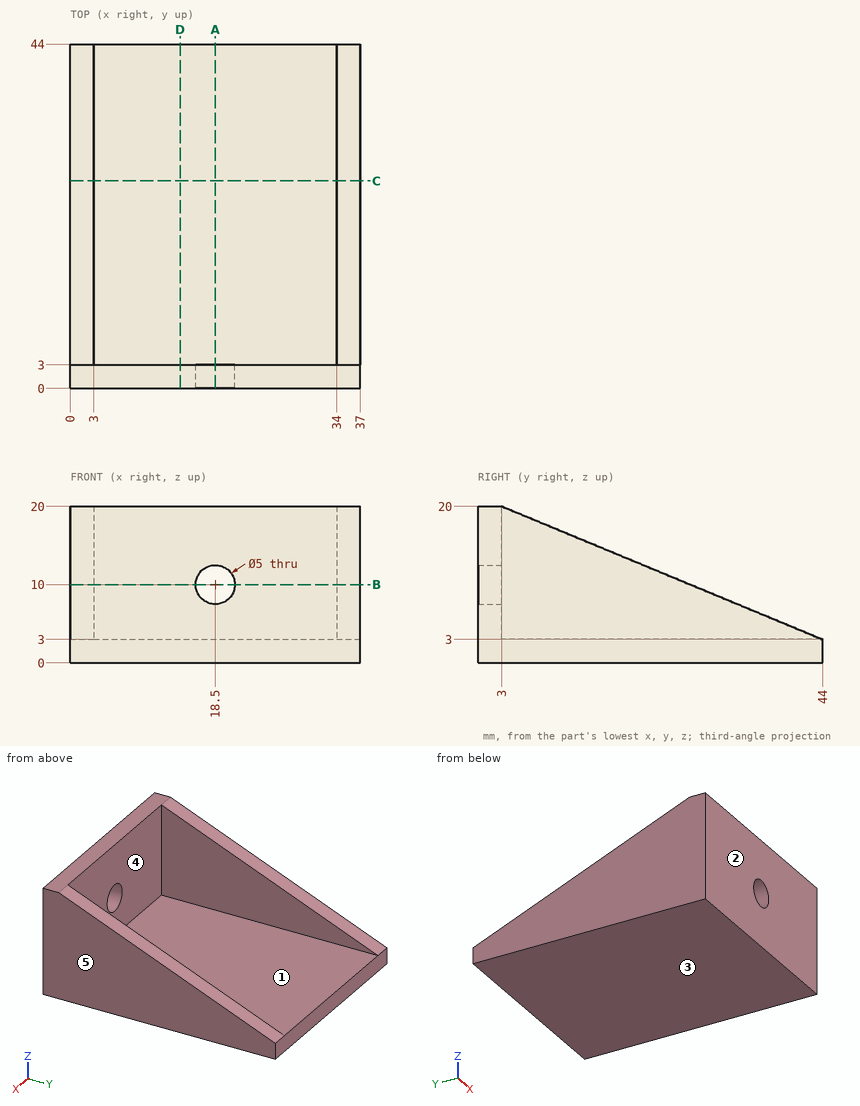
Source: three-view drawing plus pictorial views. Frame: mm from the lowest corner of the part. A direction names the side the tool comes from. Round coordinates to 2 decimals unless told otherwise and drop trailing zeros. Loops run counter-clockwise (first coordinate to the right, second up) from the corner with the lowest first, then second, coordinate; pieces in that order, holes last.
Q1. Section D-D on x = 14. Return loops of the section in (y, z), plus the area to 3 significant figures.
Q2. Section C-C on y = 26.5. Return loops of the section in (x, z), plus the area to 3 significant figures.
Q3. Section A-A on x = 18.5. Return loops of the section in (y, z), plus the area to 3 significant figures.
Q4. Section B-B on z = 10. Return loops of the section in (x, y), plus the area to 3 significant figures.
Q5. Access query for the marked faces 1 and 2. Directions: +Z, -Z, +X, -X, +Y, -Y. A direction counts if a zero-diameter tool reaches every point of the face in a straight line with its end or side. Return the directions, or none.
Q6. Pin query (flat end, axial travel): P1, Ø1.5, axis at x = 7, y = 39, coming from the +Z side; P2, Ø5, axis at x = 16, z = 15, coming from the +Y side. Return the tip coordinate at first contact, or that it passes through.
Q7. Pull-direction query (X, two-part tool) for the marked faces 3, 4 and 5; classes: released by +X, released by -X, zero draft, split by the parting line, or undercut.
Q8. Material intervals for L1, parallel to X at y = 39.5, z = 3.25; L2, parallel to Z at x = 18.5, y = 0.75; L3, parallel to Y at x = 20.5, z = 12.25, sorted ascending.
Evaluation:
1. outline: (0, 0) - (44, 0) - (44, 3) - (3, 3) - (3, 20) - (0, 20) - close
1. area: 183 mm2
2. outline: (0, 0) - (37, 0) - (37, 10.26) - (34, 10.26) - (34, 3) - (3, 3) - (3, 10.26) - (0, 10.26) - close
2. area: 155 mm2
3. outline: (0, 0) - (44, 0) - (44, 3) - (3, 3) - (3, 7.5) - (0, 7.5) - close; (0, 12.5) - (3, 12.5) - (3, 20) - (0, 20) - close
3. area: 168 mm2
4. outline: (0, 0) - (16, 0) - (16, 3) - (3, 3) - (3, 27.12) - (0, 27.12) - close; (21, 0) - (37, 0) - (37, 27.12) - (34, 27.12) - (34, 3) - (21, 3) - close
4. area: 241 mm2
5. face 1: +Z, +Y
5. face 2: +Z, -Z, +X, -X, -Y
6. P1: stops at z = 3
6. P2: stops at y = 3
7. face 3: zero draft
7. face 4: undercut
7. face 5: released by +X
8. L1: x = 0 to 3, 34 to 37
8. L2: z = 0 to 7.5, 12.5 to 20
8. L3: y = 0 to 3
